Model file for the job. Use its own axes, mm. A direction names the side the tool comes from. Coordinates: 2 decimals unless noted, no trailing zeros. Order: outer loops, then holes, each group sorted by start corner. A loop starts at its lowest first (then second) coordinate and runs counter-clockwise, first axis right, second up.
from build123d import *

# Parameters (mm, degrees)
SKETCH_1_R      = 4
SKETCH_1_R_2    = 2
EXTRUDE_1_DEPTH = 3


with BuildPart() as part:
    # 草图1 → 凸台-拉伸1 (new body)
    with BuildSketch(Plane.XY):
        Polygon((50, 44), (50, 36), (47.5, 36), (47.5, 37.5), (44.9, 37.5), (44.9, 36), (41.9, 36), (41.9, 33), (44.9, 33), (44.9, 31.5), (47.5, 31.5), (47.5, 33), (50, 33), (50, -33), (47.5, -33), (47.5, -31.5), (44.9, -31.5), (44.9, -33), (41.9, -33), (41.9, -36), (44.9, -36), (44.9, -37.5), (47.5, -37.5), (47.5, -36), (50, -36), (50, -44), (-45.00536, -44), (-45.00536, 44), align=None)
        Circle(SKETCH_1_R, mode=Mode.SUBTRACT)
        with Locations((0, -19)):
            Circle(SKETCH_1_R_2, mode=Mode.SUBTRACT)
        with Locations((-13.435028843, -13.435028843)):
            Circle(SKETCH_1_R_2, mode=Mode.SUBTRACT)
        with Locations((-19, 0)):
            Circle(SKETCH_1_R_2, mode=Mode.SUBTRACT)
        with Locations((-13.435028843, 13.435028843)):
            Circle(SKETCH_1_R_2, mode=Mode.SUBTRACT)
        with Locations((0, 19)):
            Circle(SKETCH_1_R_2, mode=Mode.SUBTRACT)
        with Locations((13.435028843, 13.435028843)):
            Circle(SKETCH_1_R_2, mode=Mode.SUBTRACT)
        with Locations((19, 0)):
            Circle(SKETCH_1_R_2, mode=Mode.SUBTRACT)
        with Locations((13.435028843, -13.435028843)):
            Circle(SKETCH_1_R_2, mode=Mode.SUBTRACT)
    extrude(amount=EXTRUDE_1_DEPTH)


solid = part.part
Q1. Cut at B-B, the plane y = 0. List the corners of the cut face in (x, z).
Established:
outline: (-45.01, 0) - (-21, 0) - (-21, 3) - (-45.01, 3) - close; (-17, 0) - (-4, 0) - (-4, 3) - (-17, 3) - close; (4, 0) - (17, 0) - (17, 3) - (4, 3) - close; (21, 0) - (50, 0) - (50, 3) - (21, 3) - close
Q2. Which spindle directions (+Z, -Z, +X, -X, +Y, -Y) get a long thin tool onto all of the face, cutting with end or side? Do faces 4 (the face through (3, -44, 1)), 5 (the face through (43, 33, 1)), 6 (the face through (46, 31.5, 1)). Say none if no direction does.
Established:
face 4: +Z, -Z, +X, -X, -Y
face 5: +Z, -Z, +X
face 6: +Z, -Z
Q3. Probe line 1 (Y direction, x = 0, z = 1.75); line 2 (Y direction, x = 13, z = 2.5); line 3 (X direction, y = -2.5, z = 1.25). List the from-to ranges inside material, lowest first.
Established:
line 1: y = -44 to -21, -17 to -4, 4 to 17, 21 to 44
line 2: y = -44 to -15.39, -11.48 to 11.48, 15.39 to 44
line 3: x = -45.01 to -3.12, 3.12 to 50
Q4. Cut at A-A, the plane x = 0. List the corners of the cut face in (y, z), plus the area to 3 significant figures.
Established:
outline: (-44, 0) - (-21, 0) - (-21, 3) - (-44, 3) - close; (-17, 0) - (-4, 0) - (-4, 3) - (-17, 3) - close; (4, 0) - (17, 0) - (17, 3) - (4, 3) - close; (21, 0) - (44, 0) - (44, 3) - (21, 3) - close
area: 216 mm2
Q5. Mould opens along X. For faces 1 (the face through (41.9, 35, 1)), 2 (the face through (3, 10, 0)), 3 (the face through (46, 37.5, 1)) say: pulls with the +X half, pulls with the -X half, needs draft (parallel to the pull), parting line crosses it, or undercut.
Established:
face 1: pulls with the +X half
face 2: needs draft
face 3: undercut
Q6. Drop flat-ended pins along their axis: P1, Ø1.5, axis at x = -23.5, y = -6.5, coming from the -Z side; P2, Ø1.5, axis at y = -34.5, z = 2, coming from the +X side. Give the stop position or say it passes through.
Established:
P1: stops at z = 0
P2: stops at x = 41.9
Q7. Cut at C-C, the plane x = 19. List the corners of the cut face in (y, z), plus the area to 3 significant figures.
Established:
outline: (-44, 0) - (-2, 0) - (-2, 3) - (-44, 3) - close; (2, 0) - (44, 0) - (44, 3) - (2, 3) - close
area: 252 mm2
Q8. Cut at D-D, the plane y = 19. List the corners of the cut face in (x, z), plus the area to 3 significant figures.
Established:
outline: (-45.01, 0) - (-2, 0) - (-2, 3) - (-45.01, 3) - close; (2, 0) - (50, 0) - (50, 3) - (2, 3) - close
area: 273 mm2
